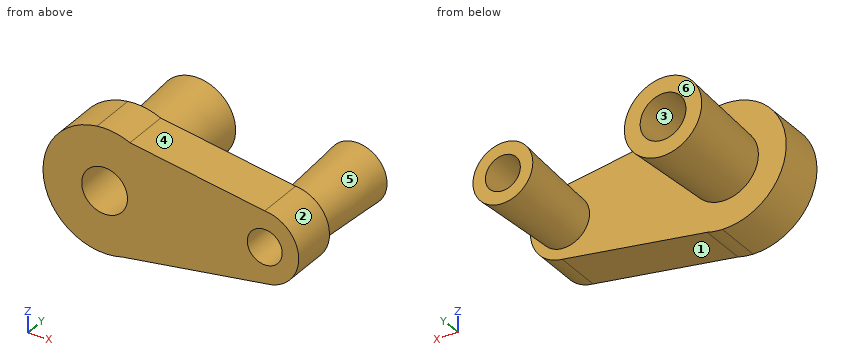
```python
from build123d import *

# Parameters (mm, degrees)
F1_DEPTH = 25.4
F2_R     = 12.5025972882
F2_R_2   = 9.5302098869
F3_DEPTH = 25.4
F4_R     = 18.4484628598
F4_R_2   = 13.6784714259
F5_DEPTH = 50.8
F5_TAPER = -3
F6_DEPTH = 50.8
F7_DEPTH = 50.8


with BuildPart() as f1:
    # F0 (on Front) → F1 (new body)
    with BuildSketch(Plane.XZ):
        with BuildLine():
            ThreePointArc((45.2668793955, -19.3830094207), (57.6364376691, -13.0022082879), (62.6026409088, 0))
            ThreePointArc((62.6026409088, 0), (57.2322577304, 13.4404517854), (44.0785706073, 19.4792658036))
            ThreePointArc((44.0785706073, 19.4792658036), (23.6039660348, -0.5961004671), (45.2668793955, -19.3830094207))
        make_face()
        with BuildLine():
            ThreePointArc((45.2668793955, -19.3830094207), (23.6039660348, -0.5961004671), (44.0785706073, 19.4792658036))
            Line((44.0785706073, 19.4792658036), (-29.5030757231, 30.6489142731))
            ThreePointArc((-29.5030757231, 30.6489142731), (-15.0912426316, 18.2411567602), (-9.7141077437, 0))
            ThreePointArc((-9.7141077437, 0), (-16.4079870718, -20.1347082672), (-33.8247665625, -32.2537135744))
            Line((-33.8247665625, -32.2537135744), (45.2668793955, -19.3830094207))
        make_face()
        with BuildLine():
            Line((-47.4639300675, 33.3753608701), (-29.5030757231, 30.6489142731))
            ThreePointArc((-29.5030757231, 30.6489142731), (-38.2959099688, 33.2479326289), (-47.4639300675, 33.3753608701))
        make_face()
        with BuildLine():
            ThreePointArc((-9.7141077437, 0), (-15.0912426316, 18.2411567602), (-29.5030757231, 30.6489142731))
            Line((-29.5030757231, 30.6489142731), (-47.4639300675, 33.3753608701))
            ThreePointArc((-47.4639300675, 33.3753608701), (-76.8661552323, -2.6627929941), (-42.1434023047, -33.6074178539))
            Line((-42.1434023047, -33.6074178539), (-33.8247665625, -32.2537135744))
            ThreePointArc((-33.8247665625, -32.2537135744), (-16.4079870718, -20.1347082672), (-9.7141077437, 0))
        make_face()
        with BuildLine():
            ThreePointArc((-42.1434023047, -33.6074178539), (-37.9415084281, -33.1921991348), (-33.8247665625, -32.2537135744))
            Line((-33.8247665625, -32.2537135744), (-42.1434023047, -33.6074178539))
        make_face()
    extrude(amount=F1_DEPTH)

    # F2 (on face) → F3 (cut)
    with BuildSketch(Plane.XZ.offset(25.4)):
        with Locations((-43.3429256082, 0)):
            Circle(F2_R)
        with Locations((44.0785706073, 0)):
            Circle(F2_R_2)
    extrude(amount=-F3_DEPTH, mode=Mode.SUBTRACT)

    # F4 (on face) → F5 (join)
    with BuildSketch(Plane(origin=(0, 0, 0), x_dir=(-1, 0, 0), z_dir=(0, 1, 0))):
        with Locations((43.3429256082, 0)):
            Circle(F4_R)
        with Locations((-44.0785706073, 0)):
            Circle(F4_R_2)
    extrude(amount=F5_DEPTH, taper=F5_TAPER)

    # F6 (cut): a face of the model
    f6_faces = [f1.faces().sort_by_distance(p)[0] for p in [
        (-43.3429256082, 0, 0),
    ]]
    extrude(f6_faces, amount=-F6_DEPTH, mode=Mode.SUBTRACT)

    # F7 (cut): a face of the model
    f7_faces = [f1.faces().sort_by_distance(p)[0] for p in [
        (44.0785706073, 0, 0),
    ]]
    extrude(f7_faces, amount=-F7_DEPTH, mode=Mode.SUBTRACT)


solid = f1.part
```
Design review of the part built by this model. Coordinates are the model's own, in mm. Face numbers are marked on the shaded views. A direction names the side the tool comes from. Coordinates: 2 decimals unless noted, no trailing zeros. Order: outer loops, then holes, each group sorted by start corner. A loop starts at its lowest first (then second) coordinate and runs counter-clockwise, first axis right, second up. Notation, with made-up numbers: M 88.25,-29 L 119.25,-29 A33 ccw 119.25,7 Z; hole C 43.25,-40 d10. An arc over 180 degrees is marked long. Answer as a JSON object with one key per item and string values. Group by question number.
1) Tool access review of the marked faces 5 and 6: name each direction out of +Z, -Z, +X, -X, +Y, -Y from which nothing blocks a thin tool from reaching the whole face with its end or side.
2) Add section B-B, the plane z = -3.5. Count the separate pieces of the cut face and the enclosed holes in it, then the cut area to 3 significant figures.
3) Add section D-D, the plane x = 15. Write out the cut boundary in (y, z), then the cut area to 3 significant figures.
4) Add section C-C, the plane y = 36.5. Write out the cut boundary in (x, z).
5) Wall thickness on L1, parallel to X at y = -8.5, z = -1.5; L2, parallel to Z at x = -43, y = 6.5; L3, parallel to Y at x = -69.5, z = 18: over which ranges is each line inside the solid? List them lowest first.
6) For pin 1 (10 mm diameter, centred on y = 6.5, z = 7.5, fed in from +X); pin 2 (8 mm diameter, centred on y = 41, z = -1.5, fed in from +X); pin 3 (10 mm diameter, centred on x = 25, y = 2.5, fed in from -Z), all flat-tipped, find the tip position at first contact; note any pin that passes through.
7) Mouldability with a two-part tool opening along Z and no side actions: class the marked faces 1, 2, 3 and 4 as pulls with the +Z half, pulls with the -Z half, needs draft (parallel to the pull), parting line crosses it, or undercut.
8) Add section A-A, the plane y = -11. Write out the cut boundary in (x, z), then the cut area to 3 significant figures.
Computed values:
{
 "1": {"face 5": "none", "face 6": "+Z, -Z, +X, -X, +Y"},
 "2": {"separate pieces": "3", "enclosed holes": "0", "area": "3,810 mm^2"},
 "3": {"outline": "M -25.4,-24.31 L 0,-24.31 L 0,23.89 L -25.4,23.89 Z", "area": "1,220 mm^2"},
 "4": {"outline": "C -43.34,0 d40.72; C 44.08,0 d31.18; hole C -43.34,0 d25.01; hole C 44.08,0 d19.06"},
 "5": {"L1": "x = -76.94 to -55.76, -30.93 to 34.67, 53.49 to 62.54", "L2": "z = -18.79 to -12.5, 12.5 to 18.79", "L3": "y = -25.4 to 0"},
 "6": {"pin 1": "stops at x = 57.91", "pin 2": "stops at x = 60.1", "pin 3": "stops at z = -23.39"},
 "7": {"face 1": "pulls with the -Z half", "face 2": "parting line crosses it", "face 3": "undercut", "face 4": "pulls with the +Z half"},
 "8": {"outline": "M -33.82,-32.25 L 45.27,-19.38 A19.5 ccw 44.08,19.48 L -29.5,30.65 A33.63 ccw long Z; hole C -43.34,0 d25.01; hole C 44.08,0 d19.06", "area": "6,190 mm^2"}
}
